Verification items for the finished model (mm, model axes). Face numbers are marked on the shaded views. A direction names the side the tool comes from. Round coordinates to 2 decimals unless told otherwise and drop trailing zeros. Loops run counter-clockwise (first coordinate to the right, second up) from the corner with the lowest first, then second, coordinate; pieces in that order, holes last.
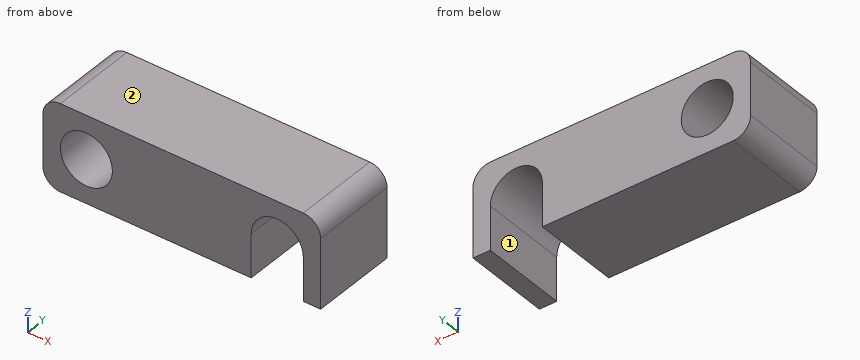
from build123d import *

# Parameters (mm, degrees)
F0_W     = 16
F0_H     = 5
F1_DEPTH = 5
F2_R     = 1.5
F3_DEPTH = 5.001
F4_R     = 1


with BuildPart() as f1:
    # F0 (on Front) → F1 (new body)
    with BuildSketch(Plane.XZ):
        with Locations((8, 2.5)):
            Rectangle(F0_W, F0_H)
    extrude(amount=F1_DEPTH)

    # F2 (on face) → F3 (cut, through all)
    with BuildSketch(Plane.XZ.offset(5)):
        with Locations((2.5, 2.5)):
            Circle(F2_R)
        with BuildLine():
            Line((15, 0), (15, 2.5))
            ThreePointArc((15, 2.5), (13.5, 4), (12, 2.5))
            Line((12, 2.5), (12, 0))
            Line((12, 0), (15, 0))
        make_face()
    extrude(amount=-F3_DEPTH, mode=Mode.SUBTRACT)

    # F4
    f4_edges = [f1.edges().sort_by_distance(p)[0] for p in [
        (0, -2.5, 0),
        (0, -2.5, 5),
        (16, -2.5, 5),
    ]]
    fillet(f4_edges, radius=F4_R)


solid = f1.part
1. Section check D-D (x = 13.5). Enter the section's corners in (y, z), then the cut area to 3 significant figures.
2. Tool access check on the marked faces 1 and 2. Record the directions out of +Z, -Z, +X, -X, +Y, -Y that give a thin tool (end or side, any length) a straight path to the whole face; none if there is none.
3. Gauge pin test, flat end, axial feed: P1, Ø1.8, axis at x = 2.5, z = 2.5, coming from the +Y side. Record the tip position at first contact, or that the pin passes through.
4. Section check B-B (x = 2.5). Enter the section's corners in (y, z).
5. Section check A-A (y = -1.85). Enter the section's corners in (x, z), then the cut area to 3 significant figures.
6. Section check C-C (z = 3.45). Enter the section's corners in (x, y), then the cut area to 3 significant figures.
7. Scan lines: L1, parallel to Z at x = 2.5, y = -1.75; L2, parallel to X at y = -0.4, z = 2.95; L3, parallel to X at y = -4, z = 3.45. Record each from-to range of solid material in increasing order.
Taken from the geometry:
1. outline: (-5, 4) - (0, 4) - (0, 5) - (-5, 5) - close
1. area: 5.00 mm2
2. face 1: -Z, +Y, -Y
2. face 2: +Z, +X, -X, +Y, -Y
3. P1: passes through
4. outline: (-5, 0) - (0, 0) - (0, 1) - (-5, 1) - close; (-5, 4) - (0, 4) - (0, 5) - (-5, 5) - close
5. outline: (0, 1) arc R1 ccw to (1, 0) - (12, 0) - (12, 2.5) arc R1.5 cw to (15, 2.5) - (15, 0) - (16, 0) - (16, 4) arc R1 ccw to (15, 5) - (1, 5) arc R1 ccw to (0, 4) - close; hole circle Ø3 at (2.5, 2.5)
5. area: 61.3 mm2
6. outline: (0, -5) - (1.34, -5) - (1.34, 0) - (0, 0) - close; (3.66, -5) - (12.34, -5) - (12.34, 0) - (3.66, 0) - close; (14.66, -5) - (16, -5) - (16, 0) - (14.66, 0) - close
6. area: 56.8 mm2
7. L1: z = 0 to 1, 4 to 5
7. L2: x = 0 to 1.07, 3.93 to 12.07, 14.93 to 16
7. L3: x = 0 to 1.34, 3.66 to 12.34, 14.66 to 16
